from build123d import *

# Parameters (mm, degrees)
LOWER_SIDE_R            = 33.25
LOWER_SIDE_R_2          = 32.45
MAIN_BODY_DEPTH         = 180
SKETCH_1_5_R            = 33.25
BOTTOM_DEPTH            = 1.2
BOTTOM_CUT_DEPTH        = 1.2
SLOPE_1_REACH           = 188.041
SLOPE_1_END_RADIUS      = 32.45
SLOPE_2_REACH           = 188.041
SLOPE_2_END_RADIUS      = 32.45
STOPPER_DEPTH           = 3
STOPPER_DRAFT           = -1
STOPPER_PROFILE_2_DEPTH = 3
STOPPER_PROFILE_2_DRAFT = -1


with BuildPart() as part:
    # lower_side → Main_body (new body)
    with BuildSketch(Plane(origin=(0, 0, 0), x_dir=(1, 0, 0), z_dir=(0, 1, 0))):
        Circle(LOWER_SIDE_R)
        Circle(LOWER_SIDE_R_2, mode=Mode.SUBTRACT)
    extrude(amount=MAIN_BODY_DEPTH)

    # Sketch 1_5 → Bottom (add)
    with BuildSketch(Plane(origin=(0, 0, 0), x_dir=(1, 0, 0), z_dir=(0, 1, 0))):
        with Locations(Location((0, 0, 0), (0, 0, 90))):
            Circle(SKETCH_1_5_R)
    extrude(amount=BOTTOM_DEPTH)

    # bottom_cut_draft → Bottom_cut (cut)
    with BuildSketch(Plane.XZ):
        with BuildLine():
            ThreePointArc((6, 12.093386622), (0, 13.5), (-6, 12.093386622))
            Line((-6, 12.093386622), (-6, -12.093386622))
            ThreePointArc((-6, -12.093386622), (0, -13.5), (6, -12.093386622))
            Line((6, -12.093386622), (6, 12.093386622))
        make_face()
        with BuildLine():
            ThreePointArc((13.5, 0), (11.472793906, 7.115124735), (6, 12.093386622))
            Line((6, 12.093386622), (6, -12.093386622))
            ThreePointArc((6, -12.093386622), (8.681837263, -10.338070503), (10.874281585, -8))
            ThreePointArc((10.874281585, -8), (11.457286814, -7.140068547), (11.972436163, -6.237849977))
            ThreePointArc((11.972436163, -6.237849977), (13.112549108, -3.211083291), (13.5, 0))
        make_face()
        with BuildLine():
            Line((-6, -12.093386622), (-6, 12.093386622))
            ThreePointArc((-6, 12.093386622), (-8.681837263, 10.338070503), (-10.874281585, 8))
            ThreePointArc((-10.874281585, 8), (-11.527291344, 7.02648947), (-12.093386622, 6))
            ThreePointArc((-12.093386622, 6), (-12.793956375, -4.308675001), (-6, -12.093386622))
        make_face()
        with BuildLine():
            Line((6, 31.5), (-6, 31.5))
            Line((-6, 31.5), (-6, 12.093386622))
            ThreePointArc((-6, 12.093386622), (0, 13.5), (6, 12.093386622))
            Line((6, 12.093386622), (6, 31.5))
        make_face()
        with BuildLine():
            ThreePointArc((6, -12.093386622), (0, -13.5), (-6, -12.093386622))
            Line((-6, -12.093386622), (-6, -31.5))
            Line((-6, -31.5), (6, -31.5))
            Line((6, -31.5), (6, -12.093386622))
        make_face()
    extrude(amount=-BOTTOM_CUT_DEPTH, mode=Mode.SUBTRACT)

    # Slope_1: up to this cylinder (the profile starts inside it)
    slope_1_end = Plane(origin=(0, 0.933333, 0), z_dir=(0, -1, 0)) * Cylinder(SLOPE_1_END_RADIUS, 441.982, mode=Mode.PRIVATE)
    # slope_draft → Slope_1 (cut, up to the surface)
    with BuildSketch(Plane.XY, mode=Mode.PRIVATE) as slope_1_sk1:
        Polygon((13.5, 1.2), (6, 1.2), (6, 0.4), align=None)
    slope_1_tool1 = extrude(slope_1_sk1.sketch, amount=SLOPE_1_REACH, mode=Mode.PRIVATE) & slope_1_end
    add(slope_1_tool1.solids().sort_by_distance((8.5, 0.933333, 0))[0], mode=Mode.SUBTRACT)

    # Slope_2: up to this cylinder (the profile starts inside it)
    slope_2_end = Plane(origin=(0, 0.933333, 0), z_dir=(0, -1, 0)) * Cylinder(SLOPE_2_END_RADIUS, 441.982, mode=Mode.PRIVATE)
    # Sketch 6_3 → Slope_2 (cut, up to the surface)
    with BuildSketch(Plane.XY, mode=Mode.PRIVATE) as slope_2_sk1:
        Polygon((-13.5, 1.2), (-6, 0.4), (-6, 1.2), align=None)
    slope_2_tool1 = extrude(slope_2_sk1.sketch, amount=-SLOPE_2_REACH, mode=Mode.PRIVATE) & slope_2_end
    add(slope_2_tool1.solids().sort_by_distance((-8.5, 0.933333, 0))[0], mode=Mode.SUBTRACT)


with BuildPart() as stopper_tool:
    # Sketch 5_3 → Stopper (with draft: the straight prism first)
    with BuildSketch(Plane.XZ):
        with BuildLine():
            ThreePointArc((11.972436163, -6.237849977), (11.457286814, -7.140068547), (10.874281585, -8))
            Line((10.874281585, -8), (32.273247435, -8))
            ThreePointArc((32.273247435, -8), (32.478394099, -7.121545951), (32.659634531, -6.237849977))
            Line((32.659634531, -6.237849977), (11.972436163, -6.237849977))
        make_face()
    extrude(amount=-STOPPER_DEPTH)
    # Stopper: the draft: its side faces are tilted about the plane it starts from
    stopper_sides = [stopper_tool.faces().sort_by_distance(p)[0] for p in [
        (11.457286814, 1.5, -7.140068547),
        (21.57376451, 1.5, -8),
        (32.478394099, 1.5, -7.121545951),
        (22.316035347, 1.5, -6.237849977),
    ]]
    draft(stopper_sides, Plane.XZ, STOPPER_DRAFT)


with BuildPart() as part_1:
    add(part.part)

    # Stopper: add stopper_tool
    add(stopper_tool.part)


with BuildPart() as stopper_profile_2_tool:
    # Sketch 5_3 → Stopper profile 2 (with draft: the straight prism first)
    with BuildSketch(Plane.XZ):
        with BuildLine():
            ThreePointArc((-12.093386622, 6), (-11.527291344, 7.02648947), (-10.874281585, 8))
            Line((-10.874281585, 8), (-32.273247435, 8))
            ThreePointArc((-32.273247435, 8), (-32.504093238, 7.003315128), (-32.704166401, 6))
            Line((-32.704166401, 6), (-12.093386622, 6))
        make_face()
    extrude(amount=-STOPPER_PROFILE_2_DEPTH)
    # Stopper profile 2: the draft: its side faces are tilted about the plane it starts from
    stopper_profile_2_sides = [stopper_profile_2_tool.faces().sort_by_distance(p)[0] for p in [
        (-32.504093238, 1.5, 7.003315128),
        (-22.398776512, 1.5, 6),
        (-11.527291344, 1.5, 7.02648947),
        (-21.57376451, 1.5, 8),
    ]]
    draft(stopper_profile_2_sides, Plane.XZ, STOPPER_PROFILE_2_DRAFT)


with BuildPart() as part_2:
    add(part_1.part)

    # Stopper profile 2: add stopper_profile_2_tool
    add(stopper_profile_2_tool.part)


solid = part_2.part
CAD build for the part. Positions are in the model's coordinates, mm. A direction names the side the tool comes from. Give positions to 0.01 mm unless a question says otherwise; leave off trailing zeros. Write each loop counter-clockwise with the first axis right and the second up, starting at its lowest first coordinate (ties: lowest second). Pieces come first, ordered by that corner, then holes. Notation, with made-up numbers: M 71,7 L 103,7 A6 cw 103,12 Z; hole C -17.5,30.5 d4. An arc over 180 degrees is marked long. Put each result on its own line as item: value. Start each with the question number.
(1) Band-saw the part on D-D, the plane x = -23. Write the cut outline in (y, z).
(2) Mould opens along Z. For faces 3 (the face through (14, 0, 0)), 4 (the face through (-4.224, 88.943, -32.174)), 5 (the face through (17.87, 88.74, -28.04)) say: +Z half, -Z half, draft (parallel to the pull), parting line (faces both ways), or undercut.
(3) Which spindle directions (+Z, -Z, +X, -X, +Y, -Y) get a long thin tool onto all of the face, cutting with end or side? Do faces 1 (the face through (9.698, 0.794, 19.265)), 2 (the face through (7, 180, 32)). Say none if no direction does.
(4) Band-saw the part on B-B, the plane z = -16. Write the cut outline in (x, y).
(5) Band-saw the part on C-C, the plane y = 109. Write the cut outline in (x, z), and give its area (3 significant figures).
(6) Flat gauge pins, fed straight in: pin 1 Ø0.5 at (x, z) = (25.5, -7.5) entering from +Y; pin 2 Ø1 at (x, y) = (-21, 72) entering from -Z; pin 3 Ø12 at (x, y) = (11, 131.5) entering from -Z; pin 4 Ø12 at (x, z) = (9, 25) entering from +Y. Where does each tip first touch, or does it go through?
(7) Probe L1, parallel to X at y = 81, z = 0; L2, parallel to Y at x = -6.5, z = 17. List the from-to ranges inside material, lowest first.
(8) Band-saw the part on A-A, the plane x = 0. Write the cut outline in (y, z).
Response values:
1. outline: M 0,-24.01 L 180,-24.01 L 180,-22.89 L 1.2,-22.89 L 1.2,6.02 L 3,6.05 L 3,7.95 L 1.2,7.98 L 1.2,22.89 L 180,22.89 L 180,24.01 L 0,24.01 Z
2. face 3: draft
2. face 4: undercut
2. face 5: parting line
3. face 1: +Y
3. face 2: +Z, -Z, +X, -X, +Y
4. outline: M -29.15,0 L -6,0 L -6,0.4 L -13.5,1.2 L -28.23,1.2 L -28.23,180 L -29.15,180 Z; M 6,0 L 29.15,0 L 29.15,180 L 28.23,180 L 28.23,1.2 L 6,1.2 Z
5. outline: C 0,0 d66.5; hole C 0,0 d64.9
5. area: 165 mm2
6. pin 1: stops at y = 3
6. pin 2: stops at z = -26.18
6. pin 3: stops at z = -32.87
6. pin 4: stops at y = 180
7. L1: x = -33.25 to -32.45, 32.45 to 33.25
7. L2: y = 0 to 1.2
8. outline: M 0,-33.25 L 180,-33.25 L 180,-32.45 L 1.2,-32.45 L 1.2,-31.5 L 0,-31.5 Z; M 0,31.5 L 1.2,31.5 L 1.2,32.45 L 180,32.45 L 180,33.25 L 0,33.25 Z
